```python
from build123d import *

# Parameters (mm, degrees)
F0_W     = 12
F0_H     = 1
F0_H_2   = 2
F1_DEPTH = 16.5
F0_W_2   = 1
F2_DEPTH = 2.4
F3_DEPTH = 6
F4_R     = 2
F5_W     = 1
F5_H     = 1
F6_DEPTH = 3.2
F5_W_2   = 4.8
F7_DEPTH = 5
F8_W     = 4.8
F8_H     = 1.8
F9_DEPTH = 1
F10_SIZE = 1


with BuildPart() as f1:
    # F0 (on Front) → F1 (new body)
    with BuildSketch(Plane.XZ):
        with Locations((0, 0.5)):
            Rectangle(F0_W, F0_H)
        with Locations((0, 2)):
            Rectangle(F0_W, F0_H_2)
    extrude(amount=-F1_DEPTH)

    # F0 (on Front) → F2 (join)
    with BuildSketch(Plane.XZ):
        with Locations((-6.5, 2)):
            Rectangle(F0_W_2, F0_H_2)
        with Locations((6.5, 2)):
            Rectangle(F0_W_2, F0_H_2)
    extrude(amount=-F2_DEPTH)

    # F0 (on Front) → F3 (join)
    with BuildSketch(Plane.XZ):
        with Locations((6.5, 0.5)):
            Rectangle(F0_W_2, F0_H)
        with Locations((-6.5, 0.5)):
            Rectangle(F0_W_2, F0_H)
    extrude(amount=-F3_DEPTH)

    # F4
    f4_edges = [f1.edges().sort_by_distance(p)[0] for p in [
        (0, 0, 3),
    ]]
    fillet(f4_edges, radius=F4_R)

    # F5 (on face) → F6 (cut)
    with BuildSketch(Plane(origin=(0, 16.5, 0), x_dir=(-1, 0, 0), z_dir=(0, 1, 0))):
        with Locations((5.5, 0.5)):
            Rectangle(F5_W, F5_H)
        with Locations((-5.5, 0.5)):
            Rectangle(F5_W, F5_H)
    extrude(amount=-F6_DEPTH, mode=Mode.SUBTRACT)

    # F5 (on face) → F7 (join)
    with BuildSketch(Plane(origin=(0, 16.5, 0), x_dir=(-1, 0, 0), z_dir=(0, 1, 0))):
        with Locations((0, 0.5)):
            Rectangle(F5_W_2, F5_H)
    extrude(amount=F7_DEPTH)

    # F8 (on face) → F9 (join)
    with BuildSketch(Plane.XY.offset(1)):
        with Locations((0, 20.6)):
            Rectangle(F8_W, F8_H)
    extrude(amount=F9_DEPTH)

    # F10
    f10_edges = [f1.edges().sort_by_distance(p)[0] for p in [
        (0, 21.5, 2),
    ]]
    chamfer(f10_edges, length=F10_SIZE)


solid = f1.part
```
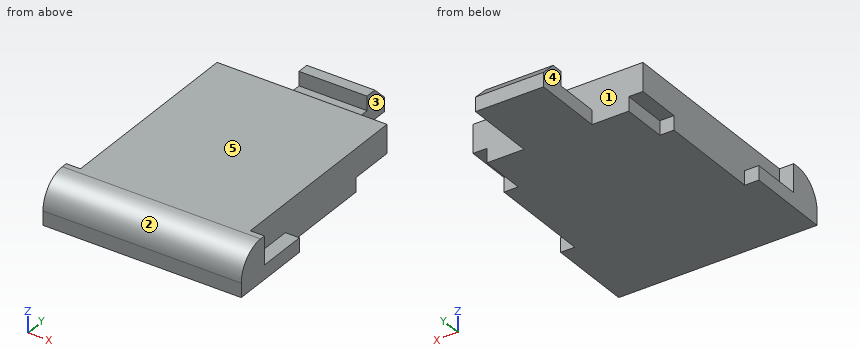
Here's how the part is built. I have some questions about the finished solid (model axes, mm). Face numbers are marked on the shaded views. A direction names the side the tool comes from. Give positions to 0.01 mm unless a question says otherwise; leave off trailing zeros. Order: outer loops, then holes, each group sorted by start corner. A loop starts at its lowest first (then second) coordinate and runs counter-clockwise, first axis right, second up. Notation, with made-up numbers: M 58,-8.5 L 79,-8.5 A31 ccw 79,22.5 Z; hole C -2.5,77.5 d11. An arc over 180 degrees is marked long. Use a Markdown table: item, result. Add a question column.
1. Suppose I cut it at B-B (x = 1). List the corners of the cut face in (y, z) for me.
2. Suppose I cut it at D-D (z = 1.55). List the corners of the cut face in (x, y) for me, and give its area (3 significant figures).
3. On a 3-axis mill with a long thin cutter (end or side, diameter ignored), from which of +Z, -Z, +X, -X, +Y, -Y can I reach the whole of each face in a straight line? I mean the marked faces 4 and 5. Say none if no direction works.
4. For pin 1 Ø0.5 at (y, z) = (14.5, 0.5) entering from -X; pin 2 Ø1.1 at (x, z) = (6.5, 1.5) entering from +Y; pin 3 Ø1 at (x, y) = (-0.5, 18) entering from +Z, each with a flat end and sliding along its axis, tell me the tip position at first contact or that it passes through.
5. Suppose I cut it at C-C (y = 4). List the corners of the cut face in (x, z) for me.
6. I need wall thicknesses on probe 1 along Y at (x, z) = (4.25, 0.65); probe 2 along X at (y, z) = (11.25, 0.55); probe 3 along Y at (x, z) = (-2, 1.1). Which ranges of each line are inside material? Lowest first, please. Write a range as from..to.
7. If we mould it in two halves opening along Y, with no side actions, what happens to the marked faces 1, 2 and 3? For each: +Y half, -Y half, draft (parallel to the pull), parting line (faces both ways), or undercut.
8. Suppose I cut it at A-A (z = 0.25). List the corners of the cut face in (x, y) for me, and give its area (3 significant figures).
Results list:
| question | item | result |
|---|---|---|
| 1 | outline | M 0,0 L 21.5,0 L 21.5,1 L 20.5,2 L 19.7,2 L 19.7,1 L 16.5,1 L 16.5,3 L 2,3 A2 ccw 0,1 Z |
| 2 | outline | M -7,0.08 L 7,0.08 L 7,2.4 L 6,2.4 L 6,16.5 L -6,16.5 L -6,2.4 L -7,2.4 Z; M -2.4,19.7 L 2.4,19.7 L 2.4,20.95 L -2.4,20.95 Z |
| 2 | area | 208 mm² |
| 3 | face 4 | +Z, -Z, -X, +Y |
| 3 | face 5 | +Z, +X, -X, +Y, -Y |
| 4 | pin 1 | stops at x = -5 |
| 4 | pin 2 | stops at y = 16.5 |
| 4 | pin 3 | stops at z = 1 |
| 5 | outline | M -7,0 L 7,0 L 7,1 L 6,1 L 6,3 L -6,3 L -6,1 L -7,1 Z |
| 6 | probe 1 | y = 0..16.5 |
| 6 | probe 2 | x = -6..6 |
| 6 | probe 3 | y = 0..16.5, 19.7..21.4 |
| 7 | face 1 | undercut |
| 7 | face 2 | -Y half |
| 7 | face 3 | draft |
| 8 | outline | M -7,0 L 7,0 L 7,6 L 6,6 L 6,13.3 L 5,13.3 L 5,16.5 L 2.4,16.5 L 2.4,21.5 L -2.4,21.5 L -2.4,16.5 L -5,16.5 L -5,13.3 L -6,13.3 L -6,6 L -7,6 Z |
| 8 | area | 228 mm² |
